Geometry check sheet. Reference: the model listing, model coordinates, mm. A direction names the side the tool comes from. Round coordinates to 2 decimals unless told otherwise and drop trailing zeros. Order: outer loops, then holes, each group sorted by start corner. A loop starts at its lowest first (then second) coordinate and runs counter-clockwise, first axis right, second up. Notation, with made-up numbers: (9.25, -13.5) - (47.25, -13.5) arc R21 ccw to (47.25, 22.5) - close; hole circle Ø9 at (9, 80). An arc over 180 degrees is marked (long way). Answer as CSV lines item,"result". Start each with the question number.
```python
from build123d import *

# Parameters (mm, degrees)
F0_R     = 10
F1_DEPTH = 5
F2_R     = 2
F3_R     = 5


with BuildPart() as f1:
    # F0 (on Top) → F1 (new body)
    with BuildSketch(Plane.XY):
        with BuildLine():
            ThreePointArc((24.792896, 14.940892), (6.554466, 26.733598), (-11.683964, 14.940892))
            ThreePointArc((-11.683964, 14.940892), (-13.445534, 6.733598), (-11.683964, -1.473696))
            ThreePointArc((-11.683964, -1.473696), (6.554466, -13.266402), (24.792896, -1.473696))
            ThreePointArc((24.792896, -1.473696), (26.109115, 2.536492), (26.554466, 6.733598))
            ThreePointArc((26.554466, 6.733598), (26.109115, 10.930704), (24.792896, 14.940892))
        make_face()
        with Locations((6.554466, 6.733598)):
            Circle(F0_R, mode=Mode.SUBTRACT)
        with BuildLine():
            Line((56.554466, 29.233598), (-43.445534, 29.233598))
            Line((-43.445534, 29.233598), (-11.683964, 14.940892))
            ThreePointArc((-11.683964, 14.940892), (6.554466, 26.733598), (24.792896, 14.940892))
            Line((24.792896, 14.940892), (56.554466, 29.233598))
        make_face()
        with BuildLine():
            ThreePointArc((24.792896, -1.473696), (6.554466, -13.266402), (-11.683964, -1.473696))
            Line((-11.683964, -1.473696), (-43.445534, -15.766402))
            Line((-43.445534, -15.766402), (56.554466, -15.766402))
            Line((56.554466, -15.766402), (24.792896, -1.473696))
        make_face()
    extrude(amount=F1_DEPTH)

    # F2
    f2_edges = [f1.edges().sort_by_distance(p)[0] for p in [
        (-43.445534, 29.233598, 2.5),
        (-43.445534, -15.766402, 2.5),
        (56.554466, -15.766402, 2.5),
        (56.554466, 29.233598, 2.5),
    ]]
    fillet(f2_edges, radius=F2_R)

    # F3
    f3_edges = [f1.edges().sort_by_distance(p)[0] for p in [
        (24.792896, 14.940892, 2.5),
        (24.792896, -1.473696, 2.5),
        (-11.683964, -1.473696, 2.5),
        (-11.683964, 14.940892, 2.5),
    ]]
    fillet(f3_edges, radius=F3_R)


solid = f1.part
```
1. Draft check along Y on faces 1 (the face through (6, -15.766, 2)), 2 (the face through (7, 29.234, 2)), 3 (the face through (49.2, 27.62, 2.54)), 4 (the face through (49.183, -14.223, 2.535)). Enter one of: released by +Y, released by -Y, zero draft, split by the parting line, or undercut.
2. Section check D-D on y = 21. Record the boundary of the cut face in (x, z).
3. Section check B-B on y = 13. Record the boundary of the cut face in (x, z).
4. Section check C-C on x = 36.5. Record the boundary of the cut face in (y, z).
5. Access from +Z, -Z, +X, -X, +Y, -Y to the whole of each face (thin tool, end or side, straight path). Record for faces 5 (the face through (6, 17, 0)), 6 (the face through (38.61, -7.69, 2.46)), 7 (the face through (-25.23, -7.57, 2.46)).
6. Thickness scan on probe 1 along Y at (x, z) = (-20.5, 3.75); probe 2 along Y at (x, z) = (-31.5, 4.2); probe 3 along X at (y, z) = (13.5, 2.35). Record the ranges inside material, lowest first.
7. Go/stop test with a flat-tipped pin: pin 1 Ø12 at (x, y) = (6.55, 6.73) entering from +Z. Record where the tip stops, or that it passes through.
8. Section check A-A on z = 1.25. Record the boundary of the cut face in (x, y), plus the area to 3 significant figures.
Numbers:
1,face 1,"released by -Y"
1,face 2,"released by +Y"
1,face 3,"undercut"
1,face 4,"undercut"
2,outline,"(-25.15, 0) - (38.26, 0) - (38.26, 5) - (-25.15, 5) - close"
3,outline,"(-12.9, 0) - (-1.24, 0) - (-1.24, 5) - (-12.9, 5) - close; (14.35, 0) - (26, 0) - (26, 5) - (14.35, 5) - close"
4,outline,"(-15.77, 0) - (-6.74, 0) - (-6.74, 5) - (-15.77, 5) - close; (20.21, 0) - (29.23, 0) - (29.23, 5) - (20.21, 5) - close"
5,face 5,"-Z, +X, -X, +Y, -Y"
5,face 6,"+Z, -Z, +X"
5,face 7,"+Z, -Z, -X"
6,probe 1,"y = -15.77 to -5.44, 18.91 to 29.23"
6,probe 2,"y = -15.77 to -10.39, 23.86 to 29.23"
6,probe 3,"x = -13 to -0.81, 13.92 to 26.11"
7,pin 1,"passes through"
8,outline,"(-34.95, -11.94) arc R2 ccw to (-34.13, -15.77) - (47.24, -15.77) arc R2 ccw to (48.06, -11.94) - (28.89, -3.32) arc R5 cw to (26.07, 2.34) arc R20 ccw to (26.55, 6.73) arc R20 ccw to (26.07, 11.13) arc R5 cw to (28.89, 16.79) - (48.06, 25.41) arc R2 ccw to (47.24, 29.23) - (-34.13, 29.23) arc R2 ccw to (-34.95, 25.41) - (-15.78, 16.79) arc R5 cw to (-12.96, 11.13) arc R20 ccw to (-12.96, 2.34) arc R5 cw to (-15.78, -3.32) - close; hole circle Ø20 at (6.55, 6.73)"
8,area,"2,240 mm2"
